Model file for the job. Use its own axes, mm. Round coordinates to 2 decimals unless told otherwise and drop trailing zeros. Order: outer loops, then holes, each group sorted by start corner. A loop starts at its lowest first (then second) coordinate and runs counter-clockwise, first axis right, second up. Notation, with made-up numbers: (63, 57) - (97, 57) arc R11 cw to (97, 78) - close; hole circle Ø8 at (1, 70). An arc over 180 degrees is marked (long way). Write item = value, one per line.
```python
from build123d import *

# Parameters (mm, degrees)
SKETCH1_W           = 107.95
SKETCH1_H           = 63.5
BOSS_EXTRUDE1_DEPTH = 3
CUT_EXTRUDE1_REACH  = 127.278
SKETCH2_W           = 12.7
SKETCH2_H           = 3
SKETCH2_W_2         = 9.525
SKETCH2_W_3         = 3
SKETCH2_H_2         = 19.05
CUT_EXTRUDE2_REACH  = 127.278


with BuildPart() as part:
    # Sketch1 → Boss-Extrude1 (new body)
    with BuildSketch(Plane.XY):
        with Locations((53.975, 31.75)):
            Rectangle(SKETCH1_W, SKETCH1_H)
    extrude(amount=BOSS_EXTRUDE1_DEPTH)

    # Sketch2 → Cut-Extrude1 (cut, up to next)
    with BuildSketch(Plane(origin=(0, 0, 0), x_dir=(-1, 0, 0), z_dir=(0, 0, -1)), mode=Mode.PRIVATE) as cut_extrude1_sk1:
        with Locations((-66.675, 1.5)):
            Rectangle(SKETCH2_W, SKETCH2_H)
    cut_extrude1_tool1 = extrude(cut_extrude1_sk1.sketch, amount=-CUT_EXTRUDE1_REACH, mode=Mode.PRIVATE) & part.part
    # Sketch2 → Cut-Extrude1 (cut, up to next)
    with BuildSketch(Plane(origin=(0, 0, 0), x_dir=(-1, 0, 0), z_dir=(0, 0, -1)), mode=Mode.PRIVATE) as cut_extrude1_sk2:
        with Locations((-17.4625, 1.5)):
            Rectangle(SKETCH2_W_2, SKETCH2_H)
    cut_extrude1_tool2 = extrude(cut_extrude1_sk2.sketch, amount=-CUT_EXTRUDE1_REACH, mode=Mode.PRIVATE) & part.part
    # Sketch2 → Cut-Extrude1 (cut, up to next)
    with BuildSketch(Plane(origin=(0, 0, 0), x_dir=(-1, 0, 0), z_dir=(0, 0, -1)), mode=Mode.PRIVATE) as cut_extrude1_sk3:
        with Locations((-90.4875, 1.5)):
            Rectangle(SKETCH2_W_2, SKETCH2_H)
    cut_extrude1_tool3 = extrude(cut_extrude1_sk3.sketch, amount=-CUT_EXTRUDE1_REACH, mode=Mode.PRIVATE) & part.part
    # Sketch2 → Cut-Extrude1 (cut, up to next)
    with BuildSketch(Plane(origin=(0, 0, 0), x_dir=(-1, 0, 0), z_dir=(0, 0, -1)), mode=Mode.PRIVATE) as cut_extrude1_sk4:
        with Locations((-41.275, 1.5)):
            Rectangle(SKETCH2_W, SKETCH2_H)
    cut_extrude1_tool4 = extrude(cut_extrude1_sk4.sketch, amount=-CUT_EXTRUDE1_REACH, mode=Mode.PRIVATE) & part.part
    # Sketch2 → Cut-Extrude1 (cut, up to next)
    with BuildSketch(Plane(origin=(0, 0, 0), x_dir=(-1, 0, 0), z_dir=(0, 0, -1)), mode=Mode.PRIVATE) as cut_extrude1_sk5:
        with Locations((-41.275, 62)):
            Rectangle(SKETCH2_W, SKETCH2_H)
    cut_extrude1_tool5 = extrude(cut_extrude1_sk5.sketch, amount=-CUT_EXTRUDE1_REACH, mode=Mode.PRIVATE) & part.part
    # Sketch2 → Cut-Extrude1 (cut, up to next)
    with BuildSketch(Plane(origin=(0, 0, 0), x_dir=(-1, 0, 0), z_dir=(0, 0, -1)), mode=Mode.PRIVATE) as cut_extrude1_sk6:
        with Locations((-66.675, 62)):
            Rectangle(SKETCH2_W, SKETCH2_H)
    cut_extrude1_tool6 = extrude(cut_extrude1_sk6.sketch, amount=-CUT_EXTRUDE1_REACH, mode=Mode.PRIVATE) & part.part
    # Sketch2 → Cut-Extrude1 (cut, up to next)
    with BuildSketch(Plane(origin=(0, 0, 0), x_dir=(-1, 0, 0), z_dir=(0, 0, -1)), mode=Mode.PRIVATE) as cut_extrude1_sk7:
        with Locations((-17.4625, 62)):
            Rectangle(SKETCH2_W_2, SKETCH2_H)
    cut_extrude1_tool7 = extrude(cut_extrude1_sk7.sketch, amount=-CUT_EXTRUDE1_REACH, mode=Mode.PRIVATE) & part.part
    # Sketch2 → Cut-Extrude1 (cut, up to next)
    with BuildSketch(Plane(origin=(0, 0, 0), x_dir=(-1, 0, 0), z_dir=(0, 0, -1)), mode=Mode.PRIVATE) as cut_extrude1_sk8:
        with Locations((-106.45, 31.75)):
            Rectangle(SKETCH2_W_3, SKETCH2_H_2)
    cut_extrude1_tool8 = extrude(cut_extrude1_sk8.sketch, amount=-CUT_EXTRUDE1_REACH, mode=Mode.PRIVATE) & part.part
    # Sketch2 → Cut-Extrude1 (cut, up to next)
    with BuildSketch(Plane(origin=(0, 0, 0), x_dir=(-1, 0, 0), z_dir=(0, 0, -1)), mode=Mode.PRIVATE) as cut_extrude1_sk9:
        with Locations((-1.5, 31.75)):
            Rectangle(SKETCH2_W_3, SKETCH2_H_2)
    cut_extrude1_tool9 = extrude(cut_extrude1_sk9.sketch, amount=-CUT_EXTRUDE1_REACH, mode=Mode.PRIVATE) & part.part
    # Sketch2 → Cut-Extrude1 (cut, up to next)
    with BuildSketch(Plane(origin=(0, 0, 0), x_dir=(-1, 0, 0), z_dir=(0, 0, -1)), mode=Mode.PRIVATE) as cut_extrude1_sk10:
        with Locations((-90.4875, 62)):
            Rectangle(SKETCH2_W_2, SKETCH2_H)
    cut_extrude1_tool10 = extrude(cut_extrude1_sk10.sketch, amount=-CUT_EXTRUDE1_REACH, mode=Mode.PRIVATE) & part.part
    add(cut_extrude1_tool1.solids().sort_by_distance((66.675, 1.5, 0))[0], mode=Mode.SUBTRACT)
    add(cut_extrude1_tool2.solids().sort_by_distance((17.4625, 1.5, 0))[0], mode=Mode.SUBTRACT)
    add(cut_extrude1_tool3.solids().sort_by_distance((90.4875, 1.5, 0))[0], mode=Mode.SUBTRACT)
    add(cut_extrude1_tool4.solids().sort_by_distance((41.275, 1.5, 0))[0], mode=Mode.SUBTRACT)
    add(cut_extrude1_tool5.solids().sort_by_distance((41.275, 62, 0))[0], mode=Mode.SUBTRACT)
    add(cut_extrude1_tool6.solids().sort_by_distance((66.675, 62, 0))[0], mode=Mode.SUBTRACT)
    add(cut_extrude1_tool7.solids().sort_by_distance((17.4625, 62, 0))[0], mode=Mode.SUBTRACT)
    add(cut_extrude1_tool8.solids().sort_by_distance((106.45, 31.75, 0))[0], mode=Mode.SUBTRACT)
    add(cut_extrude1_tool9.solids().sort_by_distance((1.5, 31.75, 0))[0], mode=Mode.SUBTRACT)
    add(cut_extrude1_tool10.solids().sort_by_distance((90.4875, 62, 0))[0], mode=Mode.SUBTRACT)

    # Sketch3 → Cut-Extrude2 (cut, up to next)
    with BuildSketch(Plane(origin=(0, 0, 0), x_dir=(-1, 0, 0), z_dir=(0, 0, -1)), mode=Mode.PRIVATE) as cut_extrude2_sk1:
        Polygon((-3, 33.2105), (-9.35, 33.2105), (-9.35, 34.9377), (-11.6868, 34.9377), (-11.6868, 33.2105), (-13.49375, 33.2105), (-13.49375, 31.75), (-13.49375, 30.2895), (-11.6868, 30.2895), (-11.6868, 28.5623), (-9.35, 28.5623), (-9.35, 30.2895), (-3, 30.2895), (-3, 31.75), align=None)
    cut_extrude2_tool1 = extrude(cut_extrude2_sk1.sketch, amount=-CUT_EXTRUDE2_REACH, mode=Mode.PRIVATE) & part.part
    # Sketch3 → Cut-Extrude2 (cut, up to next)
    with BuildSketch(Plane(origin=(0, 0, 0), x_dir=(-1, 0, 0), z_dir=(0, 0, -1)), mode=Mode.PRIVATE) as cut_extrude2_sk2:
        Polygon((-94.45625, 30.2895), (-94.45625, 31.75), (-94.45625, 33.2105), (-96.2632, 33.2105), (-96.2632, 34.9377), (-98.6, 34.9377), (-98.6, 33.2105), (-104.95, 33.2105), (-104.95, 31.75), (-104.95, 30.2895), (-98.6, 30.2895), (-98.6, 28.5623), (-96.2632, 28.5623), (-96.2632, 30.2895), align=None)
    cut_extrude2_tool2 = extrude(cut_extrude2_sk2.sketch, amount=-CUT_EXTRUDE2_REACH, mode=Mode.PRIVATE) & part.part
    add(cut_extrude2_tool1.solids().sort_by_distance((8.720382, 31.75, 0))[0], mode=Mode.SUBTRACT)
    add(cut_extrude2_tool2.solids().sort_by_distance((99.229618, 31.75, 0))[0], mode=Mode.SUBTRACT)


solid = part.part
```
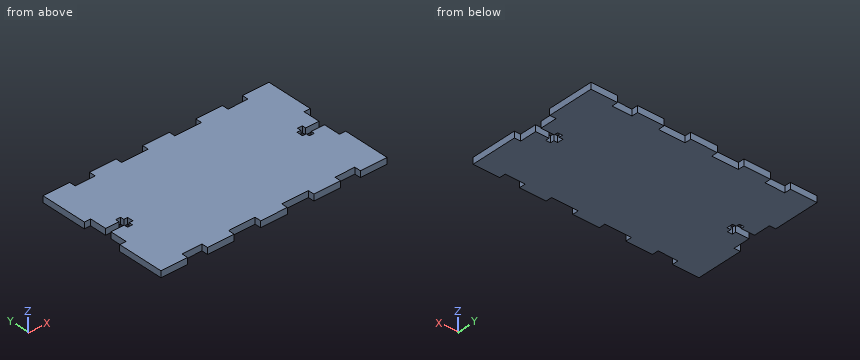
1) Wall check: line 1 along X through (y, z) = (34, 1.6); line 2 along Y through (x, z) = (102, 2.05); line 3 along Y through (x, z) = (94.5, 0.5). Give the ranges that are in metal, low to high.
Conclusion:
line_1 = 3 to 9.35, 11.69 to 96.26, 98.6 to 104.95
line_2 = 0 to 30.29, 33.21 to 63.5
line_3 = 3 to 30.29, 33.21 to 60.5
2) Cut at B-B (y = 40). Write the cut outline in (x, z), and give its area (3 significant figures).
Conclusion:
outline = (3, 0) - (104.95, 0) - (104.95, 3) - (3, 3) - close
area = 306 mm^2
3) Cut at A-A (x = 17). Write the cut outline in (y, z).
Conclusion:
outline = (3, 0) - (60.5, 0) - (60.5, 3) - (3, 3) - close
4) Flat gauge pins, fed straight in: pin 1 Ø1 at (x, z) = (38.5, 2) entering from +Y; pin 2 Ø0.5 at (y, z) = (29.5, 1.5) entering from -X. Where does each tip first touch, or does it go through?
Conclusion:
pin_1 = 60.5
pin_2 = 3
